from build123d import *

# Parameters (mm, degrees)
BOSS_EXTRU_1_DEPTH      = 6
CONG_1_R                = 3
ESQUISSE2_R             = 1
ENL_V_MAT_EXTRU_1_DEPTH = 3
CHANFREIN1_SIZE         = 3


with BuildPart() as part:
    # Esquisse1 → Boss.-Extru.1 (new body)
    with BuildSketch(Plane.XY):
        Polygon((-26.464533767, 12.30154537), (75.33141454, 71.077500491), (143.246352653, 88.745859712), (161.383942986, 21.020985262), (100.854480283, 4.809102496), (-7.520422715, -57.858487698), (-179.373873722, -57.858487698), (-179.373873722, -50.687645053), (-179.373873722, 12.291034855), align=None)
        Polygon((-25.124548608, 7.301637465), (-174.373873722, 7.291378528), (-174.373873722, -50.687645053), (-174.373873722, -52.858487698), (-8.861972593, -52.858487698), (98.923133978, 9.468053786), (155.26069475, 24.557200291), (139.700811798, 82.657041562), (77.245358051, 66.408990356), align=None, mode=Mode.SUBTRACT)
    extrude(amount=BOSS_EXTRU_1_DEPTH)

    # Congé1
    cong_1_edges = [part.edges().sort_by_distance(p)[0] for p in [
        (75.33141454, 71.077500491, 3),
        (143.246352653, 88.745859712, 3),
        (161.383942986, 21.020985262, 3),
        (100.854480283, 4.809102496, 3),
        (-7.520422715, -57.858487698, 3),
        (-179.373873722, -57.858487698, 3),
        (-179.373873722, 12.291034855, 3),
        (-26.464533767, 12.30154537, 3),
    ]]
    fillet(cong_1_edges, radius=CONG_1_R)

    # Esquisse2 → Enlèv. mat.-Extru.1 (cut)
    with BuildSketch(Plane.XY):
        with Locations((158.201617013, 22.958080812)):
            Circle(ESQUISSE2_R)
        with Locations((141.388472611, 85.534334234)):
            Circle(ESQUISSE2_R)
        with Locations((76.500226548, 68.776582274)):
            Circle(ESQUISSE2_R)
        with Locations((99.890442316, 7.071415488)):
            Circle(ESQUISSE2_R)
        with Locations((-8.172352823, -55.275906246)):
            Circle(ESQUISSE2_R)
        with Locations((-25.691359515, 9.920090126)):
            Circle(ESQUISSE2_R)
        with Locations((-176.562127678, 9.920090126)):
            Circle(ESQUISSE2_R)
        with Locations((-177.029598341, -55.275906246)):
            Circle(ESQUISSE2_R)
    extrude(amount=ENL_V_MAT_EXTRU_1_DEPTH, mode=Mode.SUBTRACT)

    # Chanfrein1
    chanfrein1_edges = [part.edges().sort_by_distance(p)[0] for p in [
        (-92.349613182, -57.858487698, 6),
        (-179.373873722, -22.78362332, 6),
        (24.605627892, 41.788942262, 6),
        (-101.821199292, 12.296365586, 6),
        (46.843967712, -26.422377988, 6),
        (129.861641055, 12.578223, 6),
        (152.312387337, 54.893729991, 6),
        (108.044083383, 79.587840046, 6),
        (-178.495266971, 11.412488494, 6),
        (75.341794938, 71.05218052, 6),
        (142.628648998, 87.685066626, 6),
        (160.307894606, 21.642410085, 6),
        (-7.547920203, -57.756003669, 6),
        (-178.495194066, -56.979808041, 6),
        (100.86445313, 4.78504518, 6),
        (-26.491925042, 12.40375087, 6),
    ]]
    chamfer(chanfrein1_edges, length=CHANFREIN1_SIZE - 0.0001)  # a hair under: the kernel refuses the full size


solid = part.part
For this review, take the finished solid that the model builds, in its own axes (mm). A direction names the side the tool comes from. Round coordinates to 2 decimals unless told otherwise and drop trailing zeros. Write each loop counter-clockwise with the first axis right and the second up, starting at its lowest first coordinate (ties: lowest second). Pieces come first, ordered by that corner, then holes. Notation, with made-up numbers: (55.25, -20.75) - (104.25, -20.75) arc R12 ccw to (104.25, -8.75) - close; hole circle Ø7 at (-32, 89). An arc over 180 degrees is marked (long way). Use a Markdown table: item, result.
Q1. The part is to be moulded in two halves that separate along X. For faces 3 (the flat face through (129.88, 14.114, 4.479)), 4 (the flat face through (108.91, 74.647, 2.958)), 5 (the flat face through (23.9, 41.38, 1.48)), say which applies: pulls with the +X half, pulls with the -X half, needs draft (parallel to the pull), parting line crosses it, or undercut.
Derived:
| item | result |
|---|---|
| face 3 | pulls with the +X half |
| face 4 | undercut |
| face 5 | pulls with the -X half |
Q2. We need section A-A (x = -100.5). Give the boundary of the cut face in (y, z).
Derived:
| item | result |
|---|---|
| outline | (-57.86, 0) - (-52.86, 0) - (-52.86, 6) - (-54.86, 6) - (-57.86, 3) - close; (7.3, 0) - (12.3, 0) - (12.3, 3) - (9.3, 6) - (7.3, 6) - close |
Q3. Clearance check with flat-ended pins moving along their axes: pin 1 (3 mm diameter, centred on x = 158.2, y = 22.96, fed in from -Z); pin 2 (1.8 mm diameter, centred on x = 99.89, y = 7.07, fed in from -Z); pin 3 (1.5 mm diameter, centred on x = -110.5, z = 1, fed in from +Y); pin 4 (3 mm diameter, centred on x = 68, z = 3.5, fed in from -Y). State where each tip first meets the part, or that it passes through.
Derived:
| item | result |
|---|---|
| pin 1 | stops at z = 0 |
| pin 2 | stops at z = 3 |
| pin 3 | stops at y = 12.3 |
| pin 4 | stops at y = -15.01 |
Q4. Machinability: for faces 1 (the flat face through (147.59, 53.2, 2.96)), 2 (the flat face through (150.77, 54.94, 4.48)), which of the approach directions +Z, -Z, +X, -X, +Y, -Y give a long, thin tool a straight path to every point of the face, cutting with its end or side? Answer none if there is none.
Derived:
| item | result |
|---|---|
| face 1 | +Z, -Z |
| face 2 | +Z, +X, +Y |
Q5. We need section C-C (y = -41). Give the boundary of the cut face in (x, z).
Derived:
| item | result |
|---|---|
| outline | (-179.37, 0) - (-174.37, 0) - (-174.37, 6) - (-176.37, 6) - (-179.37, 3) - close; (11.65, 0) - (21.63, 0) - (21.63, 3) - (15.64, 6) - (11.65, 6) - close |
Q6. We need section B-B (z = 5). Give the boundary of the cut face in (x, y).
Derived:
| item | result |
|---|---|
| outline | (-177.37, -54.86) arc R1 ccw to (-176.37, -55.86) - (-8.33, -55.86) arc R1 ccw to (-7.82, -55.72) - (99.51, 6.34) arc R5 cw to (100.72, 6.84) - (157.97, 22.18) arc R1 ccw to (158.68, 23.4) - (142.09, 85.35) arc R1 ccw to (140.87, 86.06) - (76.23, 69.24) arc R1 ccw to (75.98, 69.14) - (-24.77, 10.97) arc R5 cw to (-27.27, 10.3) - (-176.37, 10.29) arc R1 ccw to (-177.37, 9.29) - close; hole (-174.37, -52.86) - (-8.86, -52.86) - (98.92, 9.47) - (155.26, 24.56) - (139.7, 82.66) - (77.25, 66.41) - (-25.12, 7.3) - (-174.37, 7.29) - close |
Q7. Wall thickness on line 1 along Y through (x, z) = (-49, 3); line 2 along X through (y, z) = (59.5, 5.5); line 3 along X through (y, z) = (-39.5, 2.5): over which ranges is each line inside the solid? List them lowest first.
Derived:
| item | result |
|---|---|
| line 1 | y = -57.86 to -52.86, 7.3 to 12.3 |
| line 2 | x = 60.28 to 65.28, 145.9 to 148.49 |
| line 3 | x = -179.37 to -174.37, 14.24 to 24.23 |
